Drawing for the job (mm, zero at the part's lowest x, y, z). Round coordinates to 2 decimals unless told otherwise and drop trailing zeros. Write each loop counter-clockwise with the first axis right and the second up, starting at its lowest first coordinate (ties: lowest second). Pieces come first, ordered by that corner, then holes.
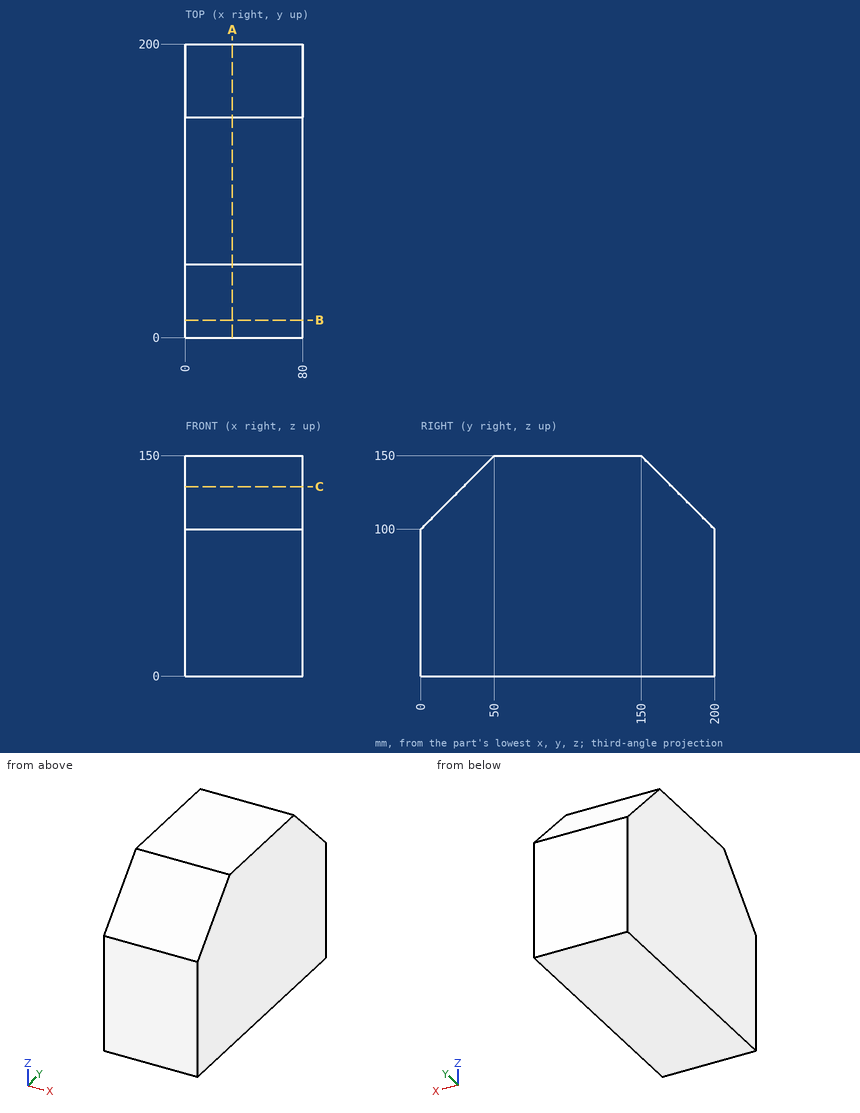
1) Wall check: probe 1 along Y at (x, z) = (60.5, 104); probe 2 along Y at (x, z) = (24, 102); probe 3 along Z at (x, y) = (53.5, 169.5). Give the ranges that are in metal, low to high.
2) Cut at B-B on y = 12. List the corners of the cut face in (x, z), and give its area (3 significant figures).
3) Flat gauge pin, fed straight in: pin 1 Ø5 at (x, y) = (56, 165.5) entering from +Z. Where does the tip first touch, or does it go through?
4) Cut at A-A on x = 32. List the corners of the cut face in (y, z).
5) Cut at C-C on z = 129. List the corners of the cut face in (x, y), and give its area (3 significant figures).
Result sheet:
1. probe 1: y = 4 to 196
1. probe 2: y = 2 to 198
1. probe 3: z = 0 to 130.5
2. outline: (0, 0) - (80, 0) - (80, 112) - (0, 112) - close
2. area: 8,960 mm2
3. pin 1: stops at z = 137
4. outline: (0, 0) - (200, 0) - (200, 100) - (150, 150) - (50, 150) - (0, 100) - close
5. outline: (0, 29) - (80, 29) - (80, 171) - (0, 171) - close
5. area: 11,400 mm2
